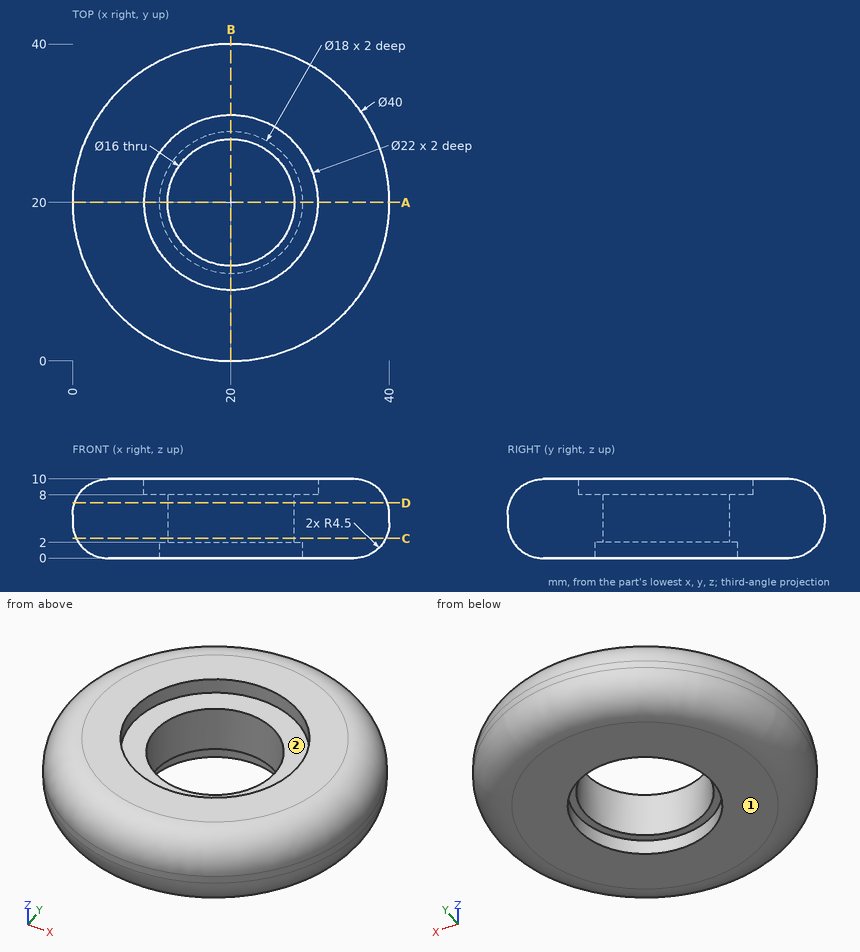
Study the drawing (mm; zero at the part's minimum x, y, z) and answer. Round coordinates to 2 decimals unless told otherwise and drop trailing zeros. Order: outer loops, then holes, each group sorted by start corner. A loop starts at its lowest first (then second) coordinate and runs counter-clockwise, first axis right, second up. Notation, with made-up numbers: M -3.5,30.25 L 27.5,30.25 A19 ccw 27.5,34.25 Z; hole C -14.5,86.5 d1. An arc over 180 degrees is marked long. One line per item, written item: value.
Q1. Straight lines are drawn through the part: line 1 (Y direction, x = 20, z = 4.4); line 2 (Y direction, x = 20.5, z = 1.5); line 3 (X direction, y = 28, z = 8.25). For each, find the intervals that lie inside material, in ascending order.
Derived:
line 1: 0 to 12, 28 to 40
line 2: 1.15 to 11.01, 28.99 to 38.85
line 3: 2.7 to 12.45, 27.55 to 37.3
Q2. Flat-ended cylindrical pins translate along their axes: pin 1 (1.5 mm diameter, centred on y = 6, z = 3, fed in from +X); pin 2 (13 mm diameter, centred on x = 20, y = 20, fed in from +Z); pin 3 (3 mm diameter, centred on y = 13, z = 2.5, fed in from -X); pin 4 (4 mm diameter, centred on y = 14, z = 8, fed in from -X). Find the tip coordinate at first contact, or state that the pin passes through.
Derived:
pin 1: x = 34.71
pin 2: through
pin 3: x = 1
pin 4: x = 0.67
Q3. Determine the mould class of the marked faces 1 and 2 for opening direction X: released by +X, released by -X, zero draft, split by the parting line, or undercut.
Derived:
face 1: zero draft
face 2: undercut
Q4. Find section D-D on z = 7. Write down the section's boundary in (x, y).
Derived:
outline: C 20,20 d39.49; hole C 20,20 d16
Q5. Find section C-C on z = 2.5. Write down the section's boundary in (x, y), then the cut area to 3 significant figures.
Derived:
outline: C 20,20 d39.06; hole C 20,20 d16
area: 997 mm²
Q6. Find section A-A on y = 20. Write down the section's boundary in (x, z).
Derived:
outline: M 0,4.5 A4.5 ccw 4.5,0 L 11,0 L 11,2 L 12,2 L 12,8 L 9,8 L 9,10 L 4.5,10 A4.5 ccw 0,5.5 Z; M 28,2 L 29,2 L 29,0 L 35.5,0 A4.5 ccw 40,4.5 L 40,5.5 A4.5 ccw 35.5,10 L 31,10 L 31,8 L 28,8 Z
